The model under review builds one solid part; all positions refer to its coordinate system, in mm. Face numbers are marked on the shaded views. A direction names the side the tool comes from. Give positions to 0.01 mm unless a question says otherwise; leave off trailing zeros. Loops run counter-clockwise (first coordinate to the right, second up) from the corner with the lowest first, then second, coordinate; pieces in that order, holes last. Notation, with made-up numbers: M 6,-37 L 52,-37 A26 ccw 52,-5 Z; hole C 61.25,-16 d11. An arc over 180 degrees is marked long. One line per item, written item: value. Start each with the question number.
Q1. To check wall thickness, follow line 1 along X through (y, z) = (1.05, 12.7); line 2 along X through (y, z) = (16, 12) (3 decimals); line 3 along X through (y, z) = (1, 12). State the ranges of each line that lie inside material, in increasing order. Write a range as from..to.
Q2. For pin 1 (5 mm diameter, centred on x = 21.5, z = 25, fed in from +Y) (3 decimals), flat-tipped, find the tip position at first contact; note if it passes through.
Q3. Mouldability with a two-part tool opening along X and no side actions: class the marked faces 3, 4 and 5 as released by +X, released by -X, zero draft, split by the parting line, or undercut.
Q4. We need section D-D on z = 35.5. Write out the cut boundary in (x, y) (3 decimals), plus the area to 3 significant figures.
Q5. For the marked faces 1 and 2, list the 3-axis set-ups (+Z, -Z, +X, -X, +Y, -Y) from which the entire face can be reached by the end or side of a thin tool; tool diameter is ignored.
Q6. We need section C-C on y = 31.75. Write out the cut boundary in (x, z) (1 decimal), plus the area to 3 significant figures.
Q7. We need section A-A on z = 19.05. Write out the cut boundary in (x, y) (1 decimal), plus the area to 3 significant figures.
Q8. We need section B-B on y = 8.5. Write out the cut boundary in (x, z) (3 decimals).
```python
from build123d import *

# Parameters (mm, degrees)
BOSS_EXTRUDE1_DEPTH = 38.1
SKETCH2_R           = 14.2875
CUT_EXTRUDE1_DEPTH  = 39.1
SKETCH3_R           = 2.4892
CUT_EXTRUDE2_DEPTH  = 4.175


with BuildPart() as part:
    # Sketch1 → Boss-Extrude1 (new body)
    with BuildSketch(Plane.XY):
        Polygon((0, 0), (0, 50.8), (3.175, 50.8), (3.175, 3.175), (34.925, 3.175), (34.925, 50.8), (38.1, 50.8), (38.1, 0), align=None)
    extrude(amount=BOSS_EXTRUDE1_DEPTH)

    # Sketch2 → Cut-Extrude1 (cut, through all)
    with BuildSketch(Plane(origin=(38.1, 0, 0), x_dir=(0, 0, -1), z_dir=(1, 0, 0))):
        with Locations((-19.05, 31.75)):
            Circle(SKETCH2_R)
    extrude(amount=-CUT_EXTRUDE1_DEPTH, mode=Mode.SUBTRACT)

    # Sketch3 → Cut-Extrude2 (cut, through all)
    with BuildSketch(Plane(origin=(0, 3.175, 0), x_dir=(1, 0, 0), z_dir=(0, 1, 0))):
        with Locations((9.525, -12.7)):
            Circle(SKETCH3_R)
        with Locations((9.525, -25.4)):
            Circle(SKETCH3_R)
        with Locations((28.575, -25.4)):
            Circle(SKETCH3_R)
        with Locations((28.575, -12.7)):
            Circle(SKETCH3_R)
    extrude(amount=-CUT_EXTRUDE2_DEPTH, mode=Mode.SUBTRACT)


solid = part.part
```
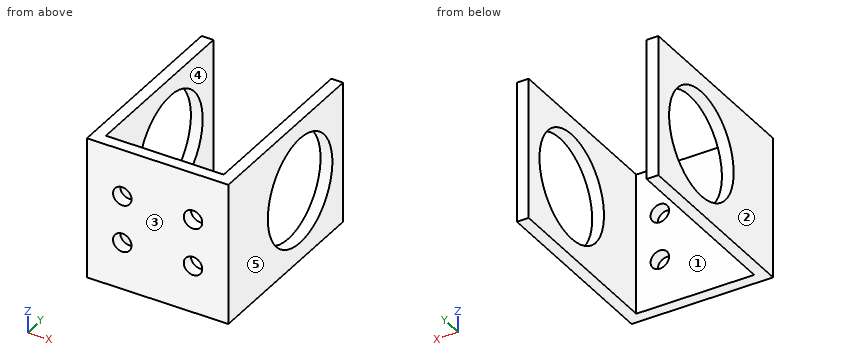
Solved:
1. line 1: 0..7.04, 12.01..26.09, 31.06..38.1
1. line 2: 0..3.175, 34.925..38.1
1. line 3: 0..7.14, 11.91..26.19, 30.96..38.1
2. pin 1: y = 3.175
3. face 3: zero draft
3. face 4: undercut
3. face 5: released by +X
4. outline: M 0,0 L 38.1,0 L 38.1,50.8 L 34.925,50.8 L 34.925,3.175 L 3.175,3.175 L 3.175,50.8 L 0,50.8 Z
4. area: 423 mm2
5. face 1: +Z, -Z, +Y
5. face 2: +Z, -Z, -X, +Y, -Y
6. outline: M 0,0 L 3.2,0 L 3.2,4.8 L 0,4.8 Z; M 0,33.3 L 3.2,33.3 L 3.2,38.1 L 0,38.1 Z; M 34.9,0 L 38.1,0 L 38.1,4.8 L 34.9,4.8 Z; M 34.9,33.3 L 38.1,33.3 L 38.1,38.1 L 34.9,38.1 Z
6. area: 60.5 mm2
7. outline: M 0,0 L 38.1,0 L 38.1,17.5 L 34.9,17.5 L 34.9,3.2 L 3.2,3.2 L 3.2,17.5 L 0,17.5 Z; M 0,46 L 3.2,46 L 3.2,50.8 L 0,50.8 Z; M 34.9,46 L 38.1,46 L 38.1,50.8 L 34.9,50.8 Z
7. area: 242 mm2
8. outline: M 0,0 L 3.175,0 L 3.175,38.1 L 0,38.1 Z; M 34.925,0 L 38.1,0 L 38.1,38.1 L 34.925,38.1 Z
